from build123d import *

# Parameters (mm, degrees)
SKETCH1_R           = 60.96
SKETCH1_R_2         = 55.88
BOSS_EXTRUDE1_DEPTH = 104.14
SKETCH2_R           = 3.3782
BOSS_EXTRUDE2_DEPTH = 6.35
CIRPATTERN1_COUNT   = 4


with BuildPart() as part:
    # Sketch1 → Boss-Extrude1 (new body)
    with BuildSketch(Plane.XY):
        Circle(SKETCH1_R)
        Circle(SKETCH1_R_2, mode=Mode.SUBTRACT)
    extrude(amount=BOSS_EXTRUDE1_DEPTH)

    # Sketch2 → Boss-Extrude2 (add)
    with BuildSketch(Plane(origin=(0, 0, 0), x_dir=(-1, 0, 0), z_dir=(0, 0, -1))):
        with BuildLine():
            Line((-48.26, 7.62), (-55.358016583, 7.62))
            ThreePointArc((-55.358016583, 7.62), (-55.88, 0), (-55.358016583, -7.62))
            Line((-55.358016583, -7.62), (-48.26, -7.62))
            ThreePointArc((-48.26, -7.62), (-40.64, 0), (-48.26, 7.62))
        make_face()
        with Locations((-48.26, 0)):
            Circle(SKETCH2_R, mode=Mode.SUBTRACT)
    boss_extrude2 = extrude(amount=-BOSS_EXTRUDE2_DEPTH)

    # CirPattern1: Boss-Extrude2 ×4 about axis
    cirpattern1_axis = Axis((0, 0, 0), (0, 0, 1))
    for i in range(1, CIRPATTERN1_COUNT):
        add(boss_extrude2.rotate(cirpattern1_axis, i * 360 / CIRPATTERN1_COUNT))


solid = part.part
Design review of the part built by this model. Coordinates are the model's own, in mm. A direction names the side the tool comes from. Give positions to 0.01 mm unless a question says otherwise; leave off trailing zeros. Order: outer loops, then holes, each group sorted by start corner. A loop starts at its lowest first (then second) coordinate and runs counter-clockwise, first axis right, second up. Notation, with made-up numbers: (-35.5, 64.5) - (-23.5, 64.5) arc R24 cw to (-23.5, 81.5) - close; hole circle Ø8 at (89, 0.25). An arc over 180 degrees is marked (long way). Write item = value, one per line. Start each with the question number.
Q1. We need section D-D on y = 24. State the section outline as (x, z) points, plus the area to 3 significant figures.
Q2. To check wall thickness, follow L1, parallel to Y at x = 0, z = 68; L2, parallel to Z at x = -50.5, y = -7; L3, parallel to X at y = -48, z = 2. State the ranges of each line that lie inside material, in increasing order. Write a range as from..to.
Q3. Clearance check with flat-ended pins moving along their axes: pin 1 Ø1 at (y, z) = (-22, 79) entering from -X; pin 2 Ø1.5 at (y, z) = (-28, 76) entering from +X; pin 3 Ø4.5 at (x, y) = (46.5, 3) entering from +Z; pin 4 Ø8 at (x, y) = (21, -44.5) entering from +Z. State where each tip first meets the part, or that it passes through.
Q4. Mouldability with a two-part tool opening along X and no side actions: class faces 1 (the face through (7.62, 52, 3)), 2 (the face through (41, 0, 0)) as released by +X, released by -X, zero draft, split by the parting line, or undercut.
Q5. We need section A-A on y = 0. State the section outline as (x, z) points, plus the area to 3 significant figures.
Q6. We need section C-C on x = 17.5. State the section outline as (y, z) points, plus the area to 3 significant figures.
Q7. Tool access review of faces 3 (the face through (-40.64, 0.17, 3.13)), 4 (the face through (0, 52, 6.35)): name each direction out of +Z, -Z, +X, -X, +Y, -Y from which nothing blocks a thin tool from reaching the whole face with its end or side.
Working result:
q1.outline = (-56.04, 0) - (-50.46, 0) - (-50.46, 104.14) - (-56.04, 104.14) - close; (50.46, 0) - (56.04, 0) - (56.04, 104.14) - (50.46, 104.14) - close
q1.area = 1,160 mm²
q2.L1 = -60.96..-55.88, 55.88..60.96
q2.L2 = 0..6.35
q2.L3 = -37.58..-28.61, -7.62..-3.37, 3.37..7.62, 28.61..37.58
q3.pin_1 = -57.04
q3.pin_2 = 54.53
q3.pin_3 = 6.35
q3.pin_4 = through
q4.face_1 = undercut
q4.face_2 = zero draft
q5.outline = (-60.96, 0) - (-51.64, 0) - (-51.64, 6.35) - (-55.88, 6.35) - (-55.88, 104.14) - (-60.96, 104.14) - close; (-44.88, 0) - (-40.64, 0) - (-40.64, 6.35) - (-44.88, 6.35) - close; (40.64, 0) - (44.88, 0) - (44.88, 6.35) - (40.64, 6.35) - close; (51.64, 0) - (60.96, 0) - (60.96, 104.14) - (55.88, 104.14) - (55.88, 6.35) - (51.64, 6.35) - close
q5.area = 1,170 mm²
q6.outline = (-58.39, 0) - (-53.07, 0) - (-53.07, 104.14) - (-58.39, 104.14) - close; (53.07, 0) - (58.39, 0) - (58.39, 104.14) - (53.07, 104.14) - close
q6.area = 1,110 mm²
q7.face_3 = +Z, -Z
q7.face_4 = +Z
